Geometry: see drawing. Coordinates: mm, zero at the bounding-box minimum. Coordinates: 2 decimals unless noted, no trailing zeros. Order: outer loops, then holes, each group sorted by start corner. A loop starts at its lowest first (then second) coordinate and runs counter-clockwise, first axis right, second up. Notation, with made-up numbers: (-34.5, 85.25) -> (-14.5, 85.25) arc R11 ccw to (-14.5, 99.25) -> close; hole circle Ø8 at (14, 33.5). An arc over 180 degrees is marked (long way). Use CSV: the item, a comma, the result in double quotes. Start each with the question number.
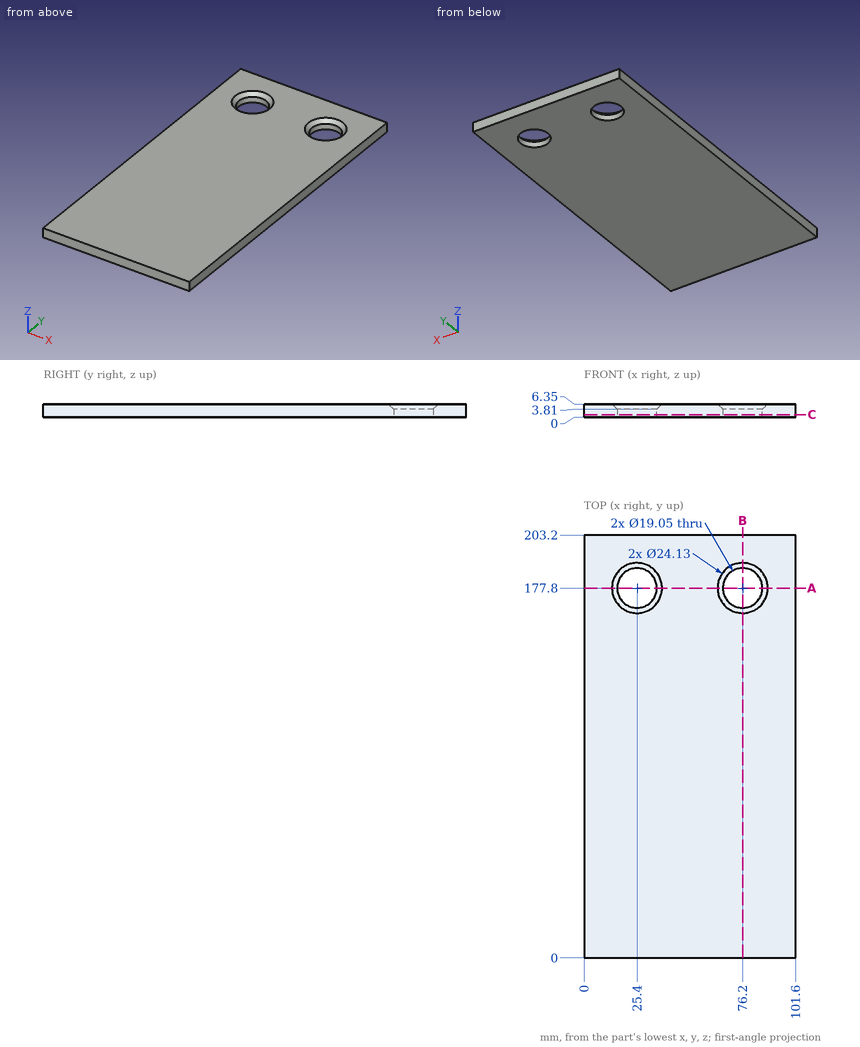
(1) First-contact query: pin 1 (5 mm diameter, centred on x = 23.5, y = 39.5, fed in from -Z); pin 2 (15 mm diameter, centred on x = 76.2, y = 177.8, fed in from +Z). Flat tips, straight axial feed; report the tip coordinate or a pass-through.
(2) Line query: line 1 (X direction, y = 177.8, z = 1.15) (3 decimals); line 2 (Y direction, x = 25.4, z = 2.7) (3 decimals); line 3 (Y direction, x = 67.5, z = 1). Output: solid intervals per line, ascending. Write a range as from..to.
(3) Section C-C (z = 1.25). Return loops of the section in (x, y) (3 decimals), then the cut area to 3 significant figures.
(4) Section A-A (y = 177.8). Return loops of the section in (x, z) (3 decimals).
(5) Section B-B (x = 76.2). Return loops of the section in (y, z) (3 decimals), then the cut area to 3 significant figures.
Check sheet entries:
1,pin 1,"stops at z = 0"
1,pin 2,"passes through"
2,line 1,"x = 0..15.875, 34.925..66.675, 85.725..101.6"
2,line 2,"y = 0..168.275, 187.325..203.2"
2,line 3,"y = 0..173.92, 181.68..203.2"
3,outline,"(0, 0) -> (101.6, 0) -> (101.6, 203.2) -> (0, 203.2) -> close; hole circle Ø19.05 at (25.4, 177.8); hole circle Ø19.05 at (76.2, 177.8)"
3,area,"20,100 mm^2"
4,outline,"(0, 0) -> (15.875, 0) -> (15.875, 3.81) -> (13.335, 6.35) -> (0, 6.35) -> close; (34.925, 0) -> (66.675, 0) -> (66.675, 3.81) -> (64.135, 6.35) -> (37.465, 6.35) -> (34.925, 3.81) -> close; (85.725, 0) -> (101.6, 0) -> (101.6, 6.35) -> (88.265, 6.35) -> (85.725, 3.81) -> close"
5,outline,"(0, 0) -> (168.275, 0) -> (168.275, 3.81) -> (165.735, 6.35) -> (0, 6.35) -> close; (187.325, 0) -> (203.2, 0) -> (203.2, 6.35) -> (189.865, 6.35) -> (187.325, 3.81) -> close"
5,area,"1,160 mm^2"
